Design review of the part built by this model. Coordinates are the model's own, in mm. Coordinates: 2 decimals unless noted, no trailing zeros. Write each loop counter-clockwise with the first axis right and the second up, starting at its lowest first coordinate (ties: lowest second). Pieces come first, ordered by that corner, then holes. Notation, with made-up numbers: (-36, 72) - (-22, 72) arc R23 cw to (-22, 99) - close; hole circle Ø3 at (10, 1.5). An arc over 180 degrees is marked (long way). Answer as a JSON object with one key per item and string values.
```python
from build123d import *

# Parameters (mm, degrees)
F0_R     = 2.75
F1_DEPTH = 4
F2_DEPTH = 23
F3_START = 23
F3_DEPTH = 4


with BuildPart() as f1:
    # F0 (on Top) → F1 (new body)
    with BuildSketch(Plane.XY):
        with BuildLine():
            Line((12.5014606537, 18.5), (12.0014606537, 0))
            Line((12.0014606537, 0), (22.2753825582, 0))
            ThreePointArc((22.2753825582, 0), (31.378069952, 5.859820993), (29.8127336093, 16.571783558))
            Line((29.8127336093, 16.571783558), (12.0014606537, 37))
            Line((12.0014606537, 37), (12.5014606537, 18.5))
        make_face()
        with Locations((22.2753825582, 10)):
            Circle(F0_R, mode=Mode.SUBTRACT)
    extrude(amount=F1_DEPTH)

    # F0 (on Top) → F2, piece 2 (join)
    with BuildSketch(Plane.XY):
        Polygon((8.5, 18.5), (8, 0), (12.0014606537, 0), (12.5014606537, 18.5), (12.0014606537, 37), (8, 37), align=None)
    extrude(amount=F2_DEPTH)



with BuildPart() as f1b:
    # F0 (on Top) → F1, piece 2 (new body)
    with BuildSketch(Plane.XY):
        with BuildLine():
            ThreePointArc((-29.8127336093, 16.571783558), (-31.378069952, 5.859820993), (-22.2753825582, 0))
            Line((-22.2753825582, 0), (-12.0014606537, 0))
            Line((-12.0014606537, 0), (-12.5014606537, 18.5))
            Line((-12.5014606537, 18.5), (-12.0014606537, 37))
            Line((-12.0014606537, 37), (-29.8127336093, 16.571783558))
        make_face()
        with Locations((-22.2753825582, 10)):
            Circle(F0_R, mode=Mode.SUBTRACT)
    extrude(amount=F1_DEPTH)

    # F0 (on Top) → F2 (join)
    with BuildSketch(Plane.XY):
        Polygon((-12.5014606537, 18.5), (-12.0014606537, 0), (-8, 0), (-8.5, 18.5), (-8, 37), (-12.0014606537, 37), align=None)
    extrude(amount=F2_DEPTH)


with BuildPart() as f1_1:
    add(f1.part)

    add(f1b.part)  # F3 merges F1b
    # F0 (on Top) → F3 (join)
    with BuildSketch(Plane.XY.offset(F3_START)):
        Polygon((-8.5, 18.5), (-8, 0), (8, 0), (8.5, 18.5), (8, 37), (-8, 37), align=None)
        Polygon((-12.5014606537, 18.5), (-12.0014606537, 0), (-8, 0), (-8.5, 18.5), (-8, 37), (-12.0014606537, 37), align=None)
        Polygon((8.5, 18.5), (8, 0), (12.0014606537, 0), (12.5014606537, 18.5), (12.0014606537, 37), (8, 37), align=None)
    extrude(amount=F3_DEPTH)


solid = f1_1.part
```
(1) The part is to be moulded in two halves that separate along X. For faces 1 (the face through (21.032, 26.643, 1.972)), 2 (the face through (17, 15, 0)), 3 (the face through (-24.3, 11.86, 1.97)), say which applies: pulls with the +X half, pulls with the -X half, needs draft (parallel to the pull), parting line crosses it, or undercut.
Solved:
{"face 1": "pulls with the +X half", "face 2": "needs draft", "face 3": "undercut"}
(2) Take a section at B-B, the plane y = 10. Write out the cut boundary in (x, z).
Solved:
{"outline": "(-32.28, 0) - (-25.03, 0) - (-25.03, 4) - (-32.28, 4) - close; (-19.53, 0) - (-8.27, 0) - (-8.27, 23) - (8.27, 23) - (8.27, 0) - (19.53, 0) - (19.53, 4) - (12.27, 4) - (12.27, 27) - (-12.27, 27) - (-12.27, 4) - (-19.53, 4) - close; (25.03, 0) - (32.28, 0) - (32.28, 4) - (25.03, 4) - close"}
(3) For pin 1 (2 mm diameter, centred on y = 22, z = 24, fed in from +X); pin 2 (2 mm diameter, centred on y = 17.5, z = 3, fed in from -X); pin 3 (16 mm diameter, centred on x = -23.5, y = 23.5, fed in from +Z); pin 4 (6 mm diameter, centred on x = 27, y = 27.5, fed in from +Z), all flat-tipped, find the tip position at first contact; note any pin that passes through.
Solved:
{"pin 1": "stops at x = 12.43", "pin 2": "stops at x = -29.87", "pin 3": "stops at z = 4", "pin 4": "passes through"}
(4) Take a section at A-A, the plane z = 19. Write out the cut boundary in (x, y).
Solved:
{"outline": "(-12.5, 18.5) - (-12, 0) - (-8, 0) - (-8.5, 18.5) - (-8, 37) - (-12, 37) - close; (8, 0) - (12, 0) - (12.5, 18.5) - (12, 37) - (8, 37) - (8.5, 18.5) - close"}
(5) To check wall thickness, follow line 1 (X direction, y = 18, z = 14.5); line 2 (Z direction, x = 17, y = 9.5); line 3 (Y direction, x = -21.5, z = 2). State the ranges of each line that lie inside material, in increasing order. Write a range as from..to.
Solved:
{"line 1": "x = -12.49..-8.49, 8.49..12.49", "line 2": "z = 0..4", "line 3": "y = 0..7.36, 12.64..26.11"}
(6) Take a section at D-D, the plane x = -3. Write out the cut boundary in (y, z).
Solved:
{"outline": "(0, 23) - (37, 23) - (37, 27) - (0, 27) - close"}
(7) Take a section at C-C, the plane y = 27. Write out the cut boundary in (x, z), and give its area (3 significant figures).
Solved:
{"outline": "(-20.72, 0) - (-8.27, 0) - (-8.27, 23) - (8.27, 23) - (8.27, 0) - (20.72, 0) - (20.72, 4) - (12.27, 4) - (12.27, 27) - (-12.27, 27) - (-12.27, 4) - (-20.72, 4) - close", "area": "350 mm^2"}
